Here's how the part is built. I have some questions about the finished solid (model axes, mm). Face numbers are marked on the shaded views. A direction names the side the tool comes from. Round coordinates to 2 decimals unless told otherwise and drop trailing zeros. Write each loop counter-clockwise with the first axis right and the second up, starting at its lowest first coordinate (ties: lowest second). Pieces come first, ordered by that corner, then holes. Notation, with made-up numbers: (54.25, -0.75) - (83.25, -0.75) arc R33 ccw to (83.25, 37.25) - close; hole circle Ø1 at (-12.5, 24). An arc over 180 degrees is marked (long way). Return JSON: item names as keys, results as strings. Group by question number.
```python
from build123d import *

# Parameters (mm, degrees)
SKETCH1_W           = 40.5
SKETCH1_H           = 24
BOSS_EXTRUDE1_DEPTH = 20.25
FILLET1_R           = 5
CUT_EXTRUDE7_DEPTH  = 1.1
FILLET2_R           = 1
SKETCH14_R          = 2.5
BOSS_EXTRUDE3_DEPTH = 16.5
SKETCH15_W          = 12.5
SKETCH15_H          = 5
CUT_EXTRUDE8_DEPTH  = 12
SKETCH17_W          = 11
SKETCH17_H          = 1.8
BOSS_EXTRUDE4_DEPTH = 11
SKETCH18_W          = 1.5
SKETCH18_H          = 0.4
CUT_EXTRUDE9_DEPTH  = 2
LPATTERN1_COUNT     = 3
LPATTERN1_PITCH     = 2.1
LPATTERN1_COL_COUNT = 3
LPATTERN1_COL_PITCH = 2.1


# Read off the part's stored shape, not the designer's step: Dome1, Dome2
with BuildPart() as part:
    # Sketch1 → Boss-Extrude1 (new, symmetric)
    with BuildSketch(Plane.XY):
        Rectangle(SKETCH1_W, SKETCH1_H)
    extrude(amount=BOSS_EXTRUDE1_DEPTH, both=True)

    # Fillet1
    fillet1_edges = [part.edges().sort_by_distance(p)[0] for p in [
        (20.25, -12, 0),
        (-20.25, -12, 0),
        (-20.25, 12, 0),
        (20.25, 12, 0),
    ]]
    fillet(fillet1_edges, radius=FILLET1_R)

    # Sketch13 → Cut-Extrude7 (cut)
    with BuildSketch(Plane.XY.offset(20.25)):
        with BuildLine():
            Line((-19.05, 7), (-19.05, -7))
            ThreePointArc((-19.05, -7), (-17.937005769, -9.687005769), (-15.25, -10.8))
            Line((-15.25, -10.8), (15.25, -10.8))
            ThreePointArc((15.25, -10.8), (17.937005769, -9.687005769), (19.05, -7))
            Line((19.05, -7), (19.05, 7))
            ThreePointArc((19.05, 7), (17.937005769, 9.687005769), (15.25, 10.8))
            Line((15.25, 10.8), (-15.25, 10.8))
            ThreePointArc((-15.25, 10.8), (-17.937005769, 9.687005769), (-19.05, 7))
        make_face()
    extrude(amount=-CUT_EXTRUDE7_DEPTH, mode=Mode.SUBTRACT)

    # Fillet2
    fillet2_edges = [part.edges().sort_by_distance(p)[0] for p in [
        (-19.05, 0, 19.15),
        (-17.937005769, 9.687005769, 19.15),
        (0, 10.8, 19.15),
        (17.937005769, 9.687005769, 19.15),
        (19.05, 0, 19.15),
        (17.937005769, -9.687005769, 19.15),
        (0, -10.8, 19.15),
        (-17.937005769, -9.687005769, 19.15),
    ]]
    fillet(fillet2_edges, radius=FILLET2_R)

    # Sketch14 → Boss-Extrude3 (add)
    with BuildSketch(Plane(origin=(0, 0, -20.25), x_dir=(-1, 0, 0), z_dir=(0, 0, -1))):
        with Locations(Location((-12, 0, 0), (0, 0, 180))):
            Circle(SKETCH14_R)
        with Locations(Location((12, 0, 0), (0, 0, 180))):
            Circle(SKETCH14_R)
    extrude(amount=BOSS_EXTRUDE3_DEPTH)

    # Dome1 outline → Dome1 (revolve)
    with BuildSketch(Plane(origin=(12, 0, 0), x_dir=(1, 0, 0), z_dir=(0, -1, 0))):
        with BuildLine():
            Line((0, -36.749999997), (0, -39.25))
            ThreePointArc((0, -39.25), (1.767766954, -38.517766952), (2.5, -36.749999997))
            Line((2.5, -36.749999997), (0, -36.749999997))
        make_face()
    revolve(axis=Axis((12, 0, 0), (0, 0, 1)))

    # Dome2 outline → Dome2 (revolve)
    with BuildSketch(Plane(origin=(-12, 0, 0), x_dir=(1, 0, 0), z_dir=(0, -1, 0))):
        with BuildLine():
            Line((0, -36.749999997), (0, -39.25))
            ThreePointArc((0, -39.25), (1.767766954, -38.517766952), (2.5, -36.749999997))
            Line((2.5, -36.749999997), (0, -36.749999997))
        make_face()
    revolve(axis=Axis((-12, 0, 0), (0, 0, 1)))

    # Sketch15 → Cut-Extrude8 (cut)
    with BuildSketch(Plane.XY.offset(19.15)):
        Rectangle(SKETCH15_W, SKETCH15_H)
    extrude(amount=-CUT_EXTRUDE8_DEPTH, mode=Mode.SUBTRACT)

    # Sketch17 → Boss-Extrude4 (add)
    with BuildSketch(Plane.XY.offset(7.15)):
        with Locations((0, -0.5)):
            Rectangle(SKETCH17_W, SKETCH17_H)
    extrude(amount=BOSS_EXTRUDE4_DEPTH)

    # Sketch18 → Cut-Extrude9 (cut)
    with BuildSketch(Plane.XY.offset(18.15)):
        with Locations((0, 0.3)):
            Rectangle(SKETCH18_W, SKETCH18_H)
    cut_extrude9 = extrude(amount=-CUT_EXTRUDE9_DEPTH, mode=Mode.SUBTRACT)

    # LPattern1: Cut-Extrude9 ×3
    with Locations(*[(i * LPATTERN1_PITCH, 0, 0) for i in range(1, LPATTERN1_COUNT)]):
        add(cut_extrude9, mode=Mode.SUBTRACT)

    # LPattern1 col: Cut-Extrude9 ×3
    with Locations(*[(-i * LPATTERN1_COL_PITCH, 0, 0) for i in range(1, LPATTERN1_COL_COUNT)]):
        add(cut_extrude9, mode=Mode.SUBTRACT)


solid = part.part
```
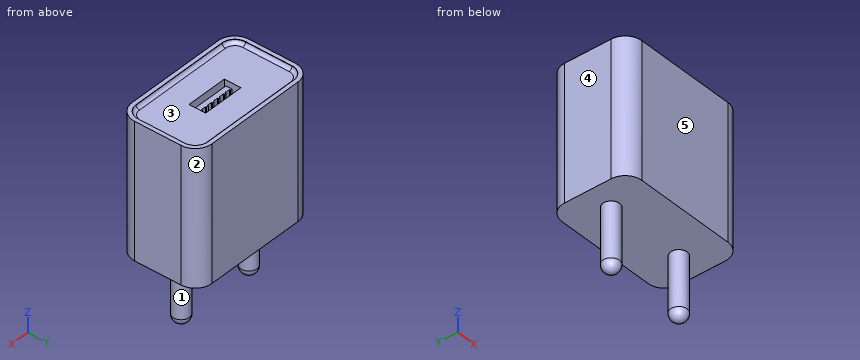
1) For the marked faces 1 and 2, which set-ups out of +Z, -Z, +X, -X, +Y, -Y let a thin tool reach every point of the face, with its end or its side?
2) Imagine slicing it at C-C (y = -4). Please give me the cut outline in (x, z).
3) If we mould it in two halves opening along X, with no side actions, what happens to the marked faces 3, 4 and 5? For each: released by +X, released by -X, zero draft, split by the parting line, or undercut.
4) Imagine slicing it at B-B (z = 3). Please give me the cut outline in (x, y), plus the area to 3 significant figures.
5) I need wall thicknesses on line 1 along Y through (x, z) = (1, 17); line 2 along Z through (x, y) = (-11.5, 8.5); line 3 along Z through (x, y) = (-4.5, -11). Which ranges of each line are inside material? Lowest first, please.
6) Imagine slicing it at D-D (x = 12). Please give me the cut outline in (y, z), plus the area to 3 significant figures.
7) Will these pins go through, and if not, where does the flat tip stop? pin 1 Ø2 at (x, y) = (-0.5, 0) entering from +Z; pin 2 Ø1.5 at (y, z) = (9.5, -8.5) entering from -X; pin 3 Ø12 at (y, z) = (-0.5, -28) entering from -X.
8) Imagine slicing it at A-A (z = 15.5). Please give me the cut outline in (x, y), plus the area to 3 significant figures.
Results found:
{
 "1": {"face 1": "-Z", "face 2": "+Z, -Z, +X, +Y"},
 "2": {"outline": "(-20.25, -20.25) - (20.25, -20.25) - (20.25, 20.25) - (19.05, 20.25) - (19.05, 20.15) arc R1 cw to (18.05, 19.15) - (-18.05, 19.15) arc R1 cw to (-19.05, 20.15) - (-19.05, 20.25) - (-20.25, 20.25) - close"},
 "3": {"face 3": "undercut", "face 4": "released by -X", "face 5": "zero draft"},
 "4": {"outline": "(-20.25, -7) arc R5 ccw to (-15.25, -12) - (15.25, -12) arc R5 ccw to (20.25, -7) - (20.25, 7) arc R5 ccw to (15.25, 12) - (-15.25, 12) arc R5 ccw to (-20.25, 7) - close", "area": "951 mm²"},
 "5": {"line 1": "y = -12 to -2.5, -1.4 to 0.4, 2.5 to 12", "line 2": "z = -20.25 to 19.15", "line 3": "z = -20.25 to 20.25"},
 "6": {"outline": "(-12, -20.25) - (-2.5, -20.25) - (-2.5, -36.75) arc R2.5 ccw to (2.5, -36.75) - (2.5, -20.25) - (12, -20.25) - (12, 20.25) - (10.8, 20.25) - (10.8, 20.15) arc R1 cw to (9.8, 19.15) - (-9.8, 19.15) arc R1 cw to (-10.8, 20.15) - (-10.8, 20.25) - (-12, 20.25) - close", "area": "1,040 mm²"},
 "7": {"pin 1": "stops at z = 18.15", "pin 2": "stops at x = -19.93", "pin 3": "stops at x = -14.5"},
 "8": {"outline": "(-20.25, -7) arc R5 ccw to (-15.25, -12) - (15.25, -12) arc R5 ccw to (20.25, -7) - (20.25, 7) arc R5 ccw to (15.25, 12) - (-15.25, 12) arc R5 ccw to (-20.25, 7) - close; (-5.5, -1.4) - (5.5, -1.4) - (5.5, 0.4) - (-5.5, 0.4) - close; hole (-6.25, -2.5) - (6.25, -2.5) - (6.25, 2.5) - (-6.25, 2.5) - close", "area": "908 mm²"}
}
